```python
from build123d import *

# Parameters (mm, degrees)
SKETCH_1_R          = 55
EXTRUDE_1_DEPTH     = 2000
SKETCH_2_R          = 50
CUT_EXTRUDE_1_DEPTH = 1900
SCALE_1_SCALE       = 0.345


with BuildPart() as part:
    # 草图1 → 凸台-拉伸1 (new body)
    with BuildSketch(Plane.XY):
        Circle(SKETCH_1_R)
    extrude(amount=EXTRUDE_1_DEPTH)

    # 草图2 → 切除-拉伸1 (cut)
    with BuildSketch(Plane.XY.offset(2000)):
        Circle(SKETCH_2_R)
    extrude(amount=-CUT_EXTRUDE_1_DEPTH, mode=Mode.SUBTRACT)


with BuildPart() as part_1:
    # 缩放比例1: scaled about (0, 0, 0)
    add(part.part.scale(SCALE_1_SCALE))


solid = part_1.part
```
CAD build for the part. Positions are in the model's coordinates, mm. A direction names the side the tool comes from. Coordinates: 2 decimals unless noted, no trailing zeros. Write each loop counter-clockwise with the first axis right and the second up, starting at its lowest first coordinate (ties: lowest second). Pieces come first, ordered by that corner, then holes. Notation, with made-up numbers: (56, -7.75) -> (99, -7.75) arc R23 cw to (99, 26.25) -> close; hole circle Ø11 at (43, 11.25). An arc over 180 degrees is marked (long way). Use CSV: the item, a comma, the result in double quotes. Start each with the question number.
Item 1: Wall check: probe 1 along Y at (x, z) = (0, 389) (3 decimals); probe 2 along X at (y, z) = (1, 290.5). Give the ranges that are in metal, low to high.
Item 2: Drop flat-ended pins along their axis: P1, Ø4, axis at x = 7.5, z = 211.5, coming from the +Y side; P2, Ø8, axis at y = 14.5, z = 190.5, coming from the -X side; P3, Ø6, axis at y = 10, z = 252.5, coming from the -X side; P4, Ø10, axis at x = -12.5, y = 8, coming from the +Z side. Give the stop position or say it passes through.
Item 3: Band-saw the part on A-A, the plane x = 0. Write the cut outline in (y, z) (3 decimals).
Item 4: Two-plate mould, pull along X, no slides. Class faces 3 (the flat face through (0, 0, 34.5)), 4 (the flat face through (4, -17, 690)), 5 (the cylindrical face through (-4.113, -18.524, 340.17)): +X half, -X half, draft (parallel to the pull), parting line (faces both ways), or undercut.
Item 5: Tool access for faces 1 (the flat face through (0, 0, 0)), 2 (the cylindrical face through (16.453, 5.181, 366.838)): list every direction of +Z, -Z, +X, -X, +Y, -Y with a clear straight run to the whole face (end or side of a thin tool).
Item 6: Band-saw the part on C-C, the plane z = 211.5. Write the cut outline in (x, y) (3 decimals).
Response values:
1,probe 1,"y = -18.975 to -17.25, 17.25 to 18.975"
1,probe 2,"x = -18.95 to -17.22, 17.22 to 18.95"
2,P1,"stops at y = 18.16"
2,P2,"stops at x = -15.81"
2,P3,"stops at x = -17.64"
2,P4,"stops at z = 690"
3,outline,"(-18.975, 0) -> (18.975, 0) -> (18.975, 690) -> (17.25, 690) -> (17.25, 34.5) -> (-17.25, 34.5) -> (-17.25, 690) -> (-18.975, 690) -> close"
4,face 3,"undercut"
4,face 4,"draft"
4,face 5,"parting line"
5,face 1,"-Z, +X, -X, +Y, -Y"
5,face 2,"+Z"
6,outline,"circle Ø37.95 at (0, 0); hole circle Ø34.5 at (0, 0)"
